Read the model definition and answer for the solid it produces. Units are mm, in the model's axes. Face numbers are marked on the shaded views. A direction names the side the tool comes from. Round coordinates to 2 decimals unless told otherwise and drop trailing zeros. Write each loop counter-clockwise with the first axis right and the second up, starting at its lowest first coordinate (ties: lowest second). Pieces come first, ordered by that corner, then holes.
Autodesk Inventor part; units mm, degrees
ref_plane "Work Plane1" through (1.525, 0, 0) normal (0, 0, 1) x (1, 0, 0)
ref_plane "YZ Plane" through (0, 0, 0) normal (1, 0, 0) x (0, 1, 0)
ref_plane "XZ Plane" through (0, 0, 0) normal (0, 1, 0) x (-1, 0, 0)
sketch "Sketch1" plane through (0, 0, 0) normal (0, 0, 1) x (1, 0, 0)
  line L0 (0, 7.7) -> (0, 5)
  line L1 (3, 5) -> (130, 5)
  line L2 (130, 5) -> (130, 0)
  line L3 (130, 0) -> (-0.6001, 0)
  line L4 (-26.7201, 0) -> (156.12, 0)
  line L5 (-0.6001, 0) -> (-0.6001, 7.7)
  line L6 (-0.6001, 7.7) -> (0, 7.7)
  line L7 (3, 5) -> (2.3864, 5)
  line L8 (2.3864, 5) -> (0, 5)
  line L9 (0, -1.54) -> (0, 9.24)
  dimension "d0" = 130
  dimension "d1" = 127
  dimension "d2" = 10
  dimension "d9" = 0.6001
  dimension "d10" = 15.4
  dimension "d13" = 0.6136
  dimension "d14" = 10
revolve "Body" add sketch "Sketch1" angle 360 about axis through (130, 0, 0) along (-1, 0, 0)
sketch "Sketch2" plane through (-0.6001, 0, 0) normal (-1, 0, 0) x (0, 0, 1)
  line L0 (0, 9.815) -> (8.5, 4.9075)
  line L1 (8.5, 4.9075) -> (8.5, -4.9075)
  line L2 (8.5, -4.9075) -> (0, -9.815)
  line L3 (0, -9.815) -> (-8.5, -4.9075)
  line L4 (-8.5, -4.9075) -> (-8.5, 4.9075)
  line L5 (-8.5, 4.9075) -> (0, 9.815)
  point P0 (0, 0)
  point P1 (0, 0)
  dimension "d11" = 17
extrude "Head" add sketch "Sketch2" along normal blind 5.8
sketch "Sketch4" plane through (0, 0, 0) normal (0, 0, 1) x (1, 0, 0)
  line L0 (-6.4001, 8.5) -> (-6.4001, 9.815)
  line L1 (-6.4001, 9.815) -> (-5.6409, 9.815)
  line L2 (-5.6409, 9.815) -> (-6.4001, 8.5)
  line L3 (-7.5601, 0) -> (0.5599, 0)
  line L4 (-0.6001, 9.815) -> (-6.4001, 9.815)
  line L5 (-6.4001, 4.9075) -> (-6.4001, 9.815)
  dimension "d5" = 30
  dimension "d19" = 17
revolve "Chamfer1" cut sketch "Sketch4" angle 360 about axis through (-10, 0, 0) along (1, 0, 0)
thread "Thread"
chamfer "Chamfer2" distance 0.6134 distance2 0.6136 1 edges at (130, -5, 0) measured on face at (130, -1.4758, -0.7745)
ref_plane "Work Plane1" through (1.525, 0, 0) normal (0, 0, 1) x (1, 0, 0)
equation "\"d0\" = NLG"
equation "\"d1\" = GEL"
equation "\"d2\" = GD"
equation "\"d10\" = SD2"
equation "\"d14\" = BDM"
equation "\"d11\" = SW"
equation "\"d3\" = KOH - SD"
equation "\"d5\" = ANG1"
equation "\"d19\" = SW0"
equation "\"d15\" = GEL"
equation "\"d6\" = -0.5 * SPD + 0.5 * GD"
equation "\"NLG\" = 130"
equation "\"GD\" = NND"
equation "\"BDM\" = NND"
equation "\"KOH\" = 6.4"
equation "\"GEL\" = 127"
equation "\"SW\" = 17"
equation "\"SW0\" = 17"
equation "\"SPD\" = NND - 1.2269 * PTC"
equation "\"SD2\" = 15.4"
equation "\"SD\" = 0.6"
equation "\"ANG1\" = 30deg"
equation "\"GAL\" = 0.61345 * PTC"
equation "\"GUL\" = 0.61345 * PTC"
equation "\"RR\" = 0"
equation "\"GD1\" = THREADDIA - 1.2269 * PTC"
equation "\"TOA\" = 30deg"
equation "\"FAWI\" = 45deg"
equation "\"PTC\" = 1"
equation "\"E0\" = 1.155 * SW"
properties part number "DIN 961 - M10 x 130" material "Steel, Mild"
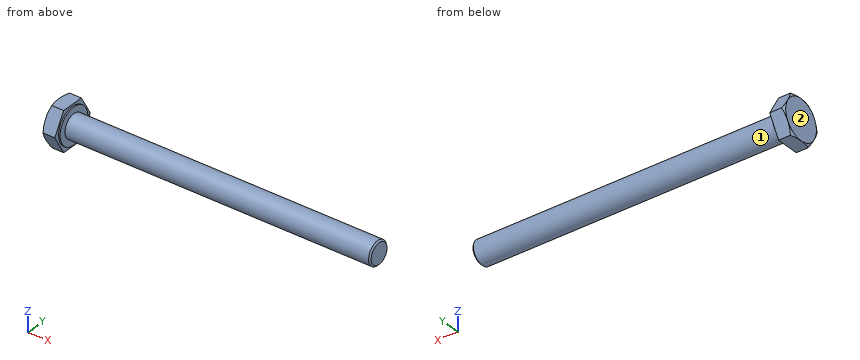
Q1. Section A-A (x = 45.5) is taken. Determine the outline of the cut face in (y, z), then the cut area to 3 significant figures.
Verdict:
outline: circle Ø10 at (0, 0)
area: 78.5 mm2
Q2. Flat-ended cylindrical pins translate along their axes: pin 1 Ø5 at (x, z) = (88.5, -3.5) entering from +Y; pin 2 Ø5 at (x, y) = (13.5, 1) entering from -Z; pin 3 Ø4 at (y, z) = (-6.5, 3.5) entering from +X. Find the tip coordinate at first contact, or state that the pin passes through.
Verdict:
pin 1: stops at y = 4.9
pin 2: stops at z = -5
pin 3: stops at x = 0
Q3. Straight lines are drawn through the part: probe 1 along Y at (x, z) = (109.5, -1); probe 2 along X at (y, z) = (2, -5); probe 3 along Z at (x, y) = (51, 0). For each, find the intervals that lie inside material, in ascending order.
Verdict:
probe 1: y = -4.9 to 4.9
probe 2: x = -6.4 to 0
probe 3: z = -5 to 5
Q4. Which of the six approach directions +Z, -Z, +X, -X, +Y, -Y give full straight-line access (tool end or side, diameter ignored) to the marked faces 1 and 2?
Verdict:
face 1: +X
face 2: +Z, -Z, -X, +Y, -Y
